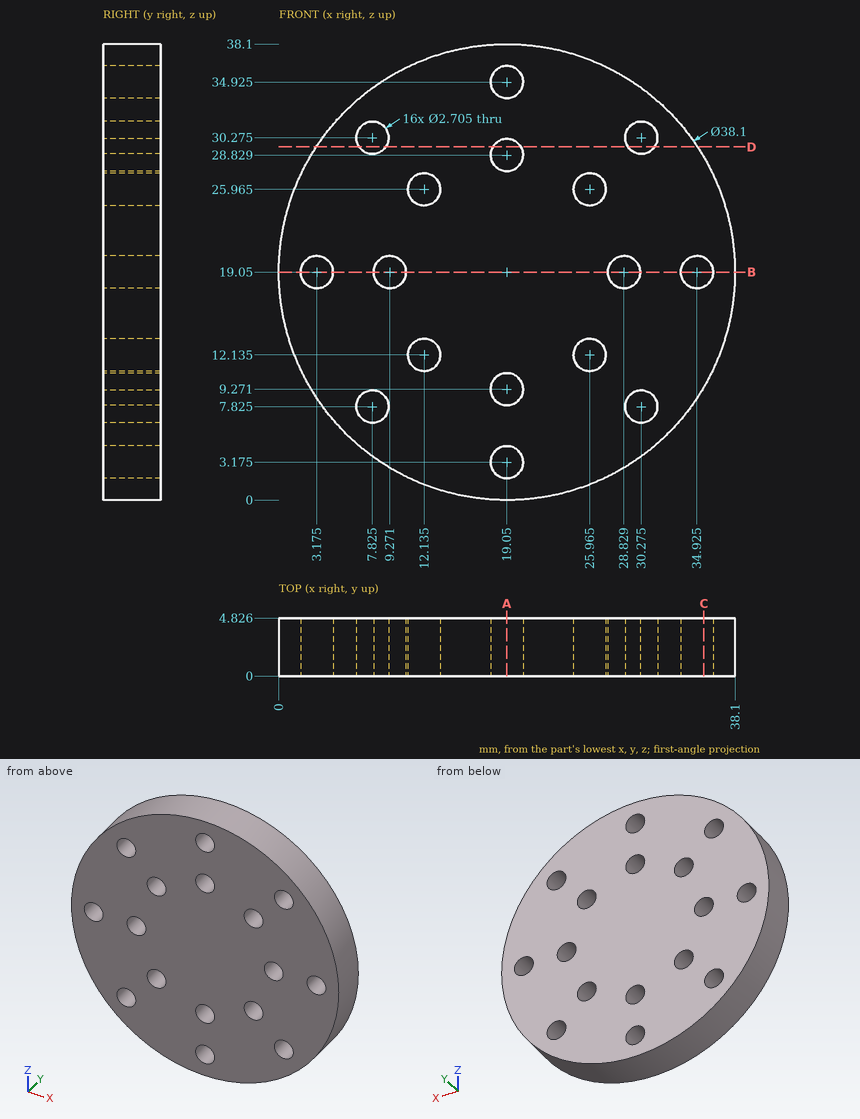
Input: dimensioned drawing with shaded views. Units: mm. Origin: part minimum x, y, z. Give positions to 0.01 mm unless a question says otherwise; leave off trailing zeros. Loops run counter-clockwise (first coordinate to the right, second up) from the corner with the lowest first, then second, coordinate; pieces in that order, holes last. Notation, with made-up numbers: (85.5, -20.5) -> (114.5, -20.5) arc R25 ccw to (114.5, -0.5) -> close; hole circle Ø8 at (-31.75, 25). An arc over 180 degrees is marked (long way). Use a Markdown table: item, result.
Q1. Section query B-B, the plane z = 19.05. Return the cut outline in (x, y).
Entries:
| item | result |
|---|---|
| outline | (0, 0) -> (1.82, 0) -> (1.82, 4.83) -> (0, 4.83) -> close; (4.53, 0) -> (7.92, 0) -> (7.92, 4.83) -> (4.53, 4.83) -> close; (10.62, 0) -> (27.48, 0) -> (27.48, 4.83) -> (10.62, 4.83) -> close; (30.18, 0) -> (33.57, 0) -> (33.57, 4.83) -> (30.18, 4.83) -> close; (36.28, 0) -> (38.1, 0) -> (38.1, 4.83) -> (36.28, 4.83) -> close |
Q2. Ray query, probe 1 along X at (y, z) = (1.35, 19); probe 2 along X at (y, z) = (4.15, 11.5). Return the intervals inside material, ascending. Write a range as from..to.
Entries:
| item | result |
|---|---|
| probe 1 | x = 0..1.82, 4.53..7.92, 10.62..27.48, 30.18..33.57, 36.28..38.1 |
| probe 2 | x = 1.56..10.94, 13.33..24.77, 27.16..36.54 |
Q3. Section query D-D, the plane z = 29.5. Return the cut outline in (x, y) (1 decimal).
Entries:
| item | result |
|---|---|
| outline | (3.1, 0) -> (6.7, 0) -> (6.7, 4.8) -> (3.1, 4.8) -> close; (8.9, 0) -> (17.9, 0) -> (17.9, 4.8) -> (8.9, 4.8) -> close; (20.2, 0) -> (29.2, 0) -> (29.2, 4.8) -> (20.2, 4.8) -> close; (31.4, 0) -> (35, 0) -> (35, 4.8) -> (31.4, 4.8) -> close |
Q4. First-contact query: P1, Ø1.6, axis at x = 12.14, z = 12.14, coming from the -Y side; P2, Ø1, axis at x = 21, y = 4.5, coming from the +Z side (1 decimal). Flat tips, straight axial feed; report the tip coordinate or a pass-through.
Entries:
| item | result |
|---|---|
| P1 | passes through |
| P2 | stops at z = 38 |
Q5. Section query C-C, the plane x = 35.5. Return the cut outline in (y, z), plus the area to 3 significant figures.
Entries:
| item | result |
|---|---|
| outline | (0, 9.44) -> (4.83, 9.44) -> (4.83, 17.83) -> (0, 17.83) -> close; (0, 20.27) -> (4.83, 20.27) -> (4.83, 28.66) -> (0, 28.66) -> close |
| area | 80.9 mm² |
Q6. Section query A-A, the plane x = 19.05. Return the cut outline in (y, z), plus the area to 3 significant figures.
Entries:
| item | result |
|---|---|
| outline | (0, 0) -> (4.83, 0) -> (4.83, 1.82) -> (0, 1.82) -> close; (0, 4.53) -> (4.83, 4.53) -> (4.83, 7.92) -> (0, 7.92) -> close; (0, 10.62) -> (4.83, 10.62) -> (4.83, 27.48) -> (0, 27.48) -> close; (0, 30.18) -> (4.83, 30.18) -> (4.83, 33.57) -> (0, 33.57) -> close; (0, 36.28) -> (4.83, 36.28) -> (4.83, 38.1) -> (0, 38.1) -> close |
| area | 132 mm² |
